```python
from build123d import *

# Parameters (mm, degrees)
BOSS_EXTRUDE1_DEPTH = 381
CUT_EXTRUDE1_REACH  = 5.175
SKETCH2_R           = 14.2875


with BuildPart() as part:
    # Sketch1 → Boss-Extrude1 (new body)
    with BuildSketch(Plane.XY):
        Polygon((3.175, 3.175), (3.175, 25.4), (0, 25.4), (0, 0), (50.8, 0), (50.8, 25.4), (47.625, 25.4), (47.625, 3.175), align=None)
    extrude(amount=BOSS_EXTRUDE1_DEPTH)

    # Sketch2 → Cut-Extrude1 (cut, up to next)
    with BuildSketch(Plane(origin=(0, 3.175, 0), x_dir=(1, 0, 0), z_dir=(0, 1, 0)), mode=Mode.PRIVATE) as cut_extrude1_sk1:
        with Locations((32.0675, -38.1)):
            Circle(SKETCH2_R)
    cut_extrude1_tool1 = extrude(cut_extrude1_sk1.sketch, amount=-CUT_EXTRUDE1_REACH, mode=Mode.PRIVATE) & part.part
    add(cut_extrude1_tool1.solids().sort_by_distance((32.0675, 3.175, 38.1))[0], mode=Mode.SUBTRACT)
    # Sketch2 → Cut-Extrude1 (cut, up to next)
    with BuildSketch(Plane(origin=(0, 3.175, 0), x_dir=(1, 0, 0), z_dir=(0, 1, 0)), mode=Mode.PRIVATE) as cut_extrude1_sk2:
        with Locations((18.7325, -69.85)):
            Circle(SKETCH2_R)
    cut_extrude1_tool2 = extrude(cut_extrude1_sk2.sketch, amount=-CUT_EXTRUDE1_REACH, mode=Mode.PRIVATE) & part.part
    add(cut_extrude1_tool2.solids().sort_by_distance((18.7325, 3.175, 69.85))[0], mode=Mode.SUBTRACT)
    # Sketch2 → Cut-Extrude1 (cut, up to next)
    with BuildSketch(Plane(origin=(0, 3.175, 0), x_dir=(1, 0, 0), z_dir=(0, 1, 0)), mode=Mode.PRIVATE) as cut_extrude1_sk3:
        with Locations((18.7325, -133.35)):
            Circle(SKETCH2_R)
    cut_extrude1_tool3 = extrude(cut_extrude1_sk3.sketch, amount=-CUT_EXTRUDE1_REACH, mode=Mode.PRIVATE) & part.part
    add(cut_extrude1_tool3.solids().sort_by_distance((18.7325, 3.175, 133.35))[0], mode=Mode.SUBTRACT)
    # Sketch2 → Cut-Extrude1 (cut, up to next)
    with BuildSketch(Plane(origin=(0, 3.175, 0), x_dir=(1, 0, 0), z_dir=(0, 1, 0)), mode=Mode.PRIVATE) as cut_extrude1_sk4:
        with Locations((32.0675, -101.6)):
            Circle(SKETCH2_R)
    cut_extrude1_tool4 = extrude(cut_extrude1_sk4.sketch, amount=-CUT_EXTRUDE1_REACH, mode=Mode.PRIVATE) & part.part
    add(cut_extrude1_tool4.solids().sort_by_distance((32.0675, 3.175, 101.6))[0], mode=Mode.SUBTRACT)
    # Sketch2 → Cut-Extrude1 (cut, up to next)
    with BuildSketch(Plane(origin=(0, 3.175, 0), x_dir=(1, 0, 0), z_dir=(0, 1, 0)), mode=Mode.PRIVATE) as cut_extrude1_sk5:
        with Locations((18.7325, -196.85)):
            Circle(SKETCH2_R)
    cut_extrude1_tool5 = extrude(cut_extrude1_sk5.sketch, amount=-CUT_EXTRUDE1_REACH, mode=Mode.PRIVATE) & part.part
    add(cut_extrude1_tool5.solids().sort_by_distance((18.7325, 3.175, 196.85))[0], mode=Mode.SUBTRACT)
    # Sketch2 → Cut-Extrude1 (cut, up to next)
    with BuildSketch(Plane(origin=(0, 3.175, 0), x_dir=(1, 0, 0), z_dir=(0, 1, 0)), mode=Mode.PRIVATE) as cut_extrude1_sk6:
        with Locations((32.0675, -165.1)):
            Circle(SKETCH2_R)
    cut_extrude1_tool6 = extrude(cut_extrude1_sk6.sketch, amount=-CUT_EXTRUDE1_REACH, mode=Mode.PRIVATE) & part.part
    add(cut_extrude1_tool6.solids().sort_by_distance((32.0675, 3.175, 165.1))[0], mode=Mode.SUBTRACT)
    # Sketch2 → Cut-Extrude1 (cut, up to next)
    with BuildSketch(Plane(origin=(0, 3.175, 0), x_dir=(1, 0, 0), z_dir=(0, 1, 0)), mode=Mode.PRIVATE) as cut_extrude1_sk7:
        with Locations((18.7325, -260.35)):
            Circle(SKETCH2_R)
    cut_extrude1_tool7 = extrude(cut_extrude1_sk7.sketch, amount=-CUT_EXTRUDE1_REACH, mode=Mode.PRIVATE) & part.part
    add(cut_extrude1_tool7.solids().sort_by_distance((18.7325, 3.175, 260.35))[0], mode=Mode.SUBTRACT)
    # Sketch2 → Cut-Extrude1 (cut, up to next)
    with BuildSketch(Plane(origin=(0, 3.175, 0), x_dir=(1, 0, 0), z_dir=(0, 1, 0)), mode=Mode.PRIVATE) as cut_extrude1_sk8:
        with Locations((32.0675, -228.6)):
            Circle(SKETCH2_R)
    cut_extrude1_tool8 = extrude(cut_extrude1_sk8.sketch, amount=-CUT_EXTRUDE1_REACH, mode=Mode.PRIVATE) & part.part
    add(cut_extrude1_tool8.solids().sort_by_distance((32.0675, 3.175, 228.6))[0], mode=Mode.SUBTRACT)
    # Sketch2 → Cut-Extrude1 (cut, up to next)
    with BuildSketch(Plane(origin=(0, 3.175, 0), x_dir=(1, 0, 0), z_dir=(0, 1, 0)), mode=Mode.PRIVATE) as cut_extrude1_sk9:
        with Locations((18.7325, -323.85)):
            Circle(SKETCH2_R)
    cut_extrude1_tool9 = extrude(cut_extrude1_sk9.sketch, amount=-CUT_EXTRUDE1_REACH, mode=Mode.PRIVATE) & part.part
    add(cut_extrude1_tool9.solids().sort_by_distance((18.7325, 3.175, 323.85))[0], mode=Mode.SUBTRACT)
    # Sketch2 → Cut-Extrude1 (cut, up to next)
    with BuildSketch(Plane(origin=(0, 3.175, 0), x_dir=(1, 0, 0), z_dir=(0, 1, 0)), mode=Mode.PRIVATE) as cut_extrude1_sk10:
        with Locations((32.0675, -292.1)):
            Circle(SKETCH2_R)
    cut_extrude1_tool10 = extrude(cut_extrude1_sk10.sketch, amount=-CUT_EXTRUDE1_REACH, mode=Mode.PRIVATE) & part.part
    add(cut_extrude1_tool10.solids().sort_by_distance((32.0675, 3.175, 292.1))[0], mode=Mode.SUBTRACT)


solid = part.part
```
Could you check a few things on this model? Use its own coordinates, in mm. A direction names the side the tool comes from. Round coordinates to 2 decimals unless told otherwise and drop trailing zeros. Loops run counter-clockwise (first coordinate to the right, second up) from the corner with the lowest first, then second, coordinate; pieces in that order, holes last. Notation, with made-up numbers: (-2, 6) - (30, 6) arc R17 cw to (30, 25) - close; hole circle Ø5 at (65, 76.5). An arc over 180 degrees is marked (long way). Answer in a Markdown table with one row per item. Add a question column.
(1) If we mould it in two halves opening along X, with no side actions, what happens to faces 1 (the face through (16.873, 1.61, 309.684)), 2 (the face through (50.8, 13, 188)), 3 (the face through (7.39, 1.61, 269.04)), 4 (the face through (27, 2, 381))? For each: pulls with the +X half, pulls with the -X half, needs draft (parallel to the pull), parting line crosses it, or undercut.
(2) If we section it at A-A (z = 38.1): Please give me the cut outline in (x, y) (3 decimals).
(3) For faces 5 (the face through (31, 3.175, 188)), 6 (the face through (15.64, 1.61, 210.8)), which set-ups out of +Z, -Z, +X, -X, +Y, -Y let a thin tool reach every point of the face, with its end or its side?
(4) I need wall thicknesses on line 1 along X through (y, z) = (2.25, 260.35) (3 decimals); line 2 along X through (y, z) = (9, 257.5) (3 decimals); line 3 along Y through (x, z) = (6.5, 228.5) (3 decimals). Which ranges of each line are inside material? Lowest first, please.
(5) If we section it at B-B (y = 22): Please give me the cut outline in (x, z) (3 decimals).
(6) If we section it at D-D (z = 313.5): Please give me the cut outline in (x, y) (3 decimals).
(7) If we section it at C-C (x = 14): Please give me the cut outline in (y, z) (3 decimals).
(8) I'm going to push a flat-ended pin straight in: pin 1 (13.5 mm diameter, centred on x = 32, z = 123.5, fed in from +Y) (3 decimals). Where does the tip first touch, or does it pass through?
Model answer:
| question | item | result |
|---|---|---|
| 1 | face 1 | undercut |
| 1 | face 2 | pulls with the +X half |
| 1 | face 3 | undercut |
| 1 | face 4 | needs draft |
| 2 | outline | (0, 0) - (17.78, 0) - (17.78, 3.175) - (3.175, 3.175) - (3.175, 25.4) - (0, 25.4) - close; (46.355, 0) - (50.8, 0) - (50.8, 25.4) - (47.625, 25.4) - (47.625, 3.175) - (46.355, 3.175) - close |
| 3 | face 5 | +Z, -Z, +Y |
| 3 | face 6 | +Y, -Y |
| 4 | line 1 | x = 0 to 4.445, 33.02 to 50.8 |
| 4 | line 2 | x = 0 to 3.175, 47.625 to 50.8 |
| 4 | line 3 | y = 0 to 3.175 |
| 5 | outline | (0, 0) - (3.175, 0) - (3.175, 381) - (0, 381) - close; (47.625, 0) - (50.8, 0) - (50.8, 381) - (47.625, 381) - close |
| 6 | outline | (0, 0) - (8.883, 0) - (8.883, 3.175) - (3.175, 3.175) - (3.175, 25.4) - (0, 25.4) - close; (28.582, 0) - (50.8, 0) - (50.8, 25.4) - (47.625, 25.4) - (47.625, 3.175) - (28.582, 3.175) - close |
| 7 | outline | (0, 0) - (3.175, 0) - (3.175, 56.369) - (0, 56.369) - close; (0, 83.331) - (3.175, 83.331) - (3.175, 119.869) - (0, 119.869) - close; (0, 146.831) - (3.175, 146.831) - (3.175, 183.369) - (0, 183.369) - close; (0, 210.331) - (3.175, 210.331) - (3.175, 246.869) - (0, 246.869) - close; (0, 273.831) - (3.175, 273.831) - (3.175, 310.369) - (0, 310.369) - close; (0, 337.331) - (3.175, 337.331) - (3.175, 381) - (0, 381) - close |
| 8 | pin 1 | stops at y = 3.175 |
